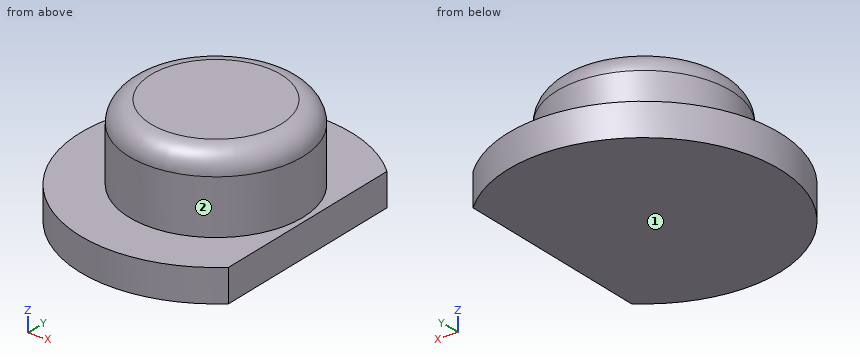
```python
from build123d import *

# Parameters (mm, degrees)
BOX116_W          = 10
BOX116_H          = 10
BOX116_DEPTH      = 10
CYLINDER019_R     = 4
CYLINDER019_DEPTH = 5
FILLET003_R       = 1
CYLINDER018_R     = 6.25
CYLINDER018_DEPTH = 1.5


with BuildPart() as cube106:
    # Box116 → Box116 (new body)
    with BuildSketch(Plane(origin=(117.3, 9, 0), x_dir=(1, 0, 0), z_dir=(0, 0, 1))):
        with Locations((5, 5)):
            Rectangle(BOX116_W, BOX116_H)
    extrude(amount=BOX116_DEPTH)


with BuildPart() as obj1:
    # Cylinder019 → Cylinder019 (new body)
    with BuildSketch(Plane(origin=(131.07, 14, 6.3), x_dir=(1, 0, 0), z_dir=(0, 0, 1))):
        Circle(CYLINDER019_R)
    extrude(amount=CYLINDER019_DEPTH)

    # Fillet003
    fillet003_edges = [obj1.edges().sort_by_distance(p)[0] for p in [
        (127.07, 14, 11.3),
    ]]
    fillet(fillet003_edges, radius=FILLET003_R)


with BuildPart() as cut072:
    # Cylinder018 → Cylinder018 (new body)
    with BuildSketch(Plane(origin=(131.07, 14, 6.3), x_dir=(1, 0, 0), z_dir=(0, 0, 1))):
        Circle(CYLINDER018_R)
    extrude(amount=CYLINDER018_DEPTH)

    # Fusion014: union obj1
    add(obj1.part)


with BuildPart() as cut072_1:
    # Fusion014 placement: moved
    add(cut072.part.moved(Location((-18, 0, 0))))

    # Cut072: cut Cube106
    add(cube106.part, mode=Mode.SUBTRACT)


solid = cut072_1.part
```
Read the model definition and answer for the solid it produces. Units are mm, in the model's axes. Face numbers are marked on the shaded views. A direction names the side the tool comes from. Coordinates: 2 decimals unless noted, no trailing zeros. Loops run counter-clockwise (first coordinate to the right, second up) from the corner with the lowest first, then second, coordinate; pieces in that order, holes last. Notation, with made-up numbers: (10, 52.25) -> (34, 52.25) arc R15 ccw to (34, 70.25) -> close; hole circle Ø10 at (7, 69). An arc over 180 degrees is marked (long way). Return JSON: item names as keys, results as strings.
Item 1: Find the intervals of material crossed by probe 1 along Z at (x, y) = (110.5, 17.75); probe 2 along Y at (x, z) = (116.5, 10.2); probe 3 along X at (y, z) = (18.5, 7.6), in increasing order.
Answers:
{"probe 1": "z = 6.3 to 7.8", "probe 2": "y = 11.94 to 16.06", "probe 3": "x = 108.73 to 117.3"}
Item 2: Find section D-D (y = 18.25). Determine the outline of the cut face in (x, z), plus the area to 3 significant figures.
Answers:
{"outline": "(108.49, 6.3) -> (117.3, 6.3) -> (117.3, 7.8) -> (108.49, 7.8) -> close", "area": "13.2 mm2"}
Item 3: Find section A-A (y = 14). Determine the outline of the cut face in (x, z).
Answers:
{"outline": "(106.82, 6.3) -> (117.3, 6.3) -> (117.3, 7.8) -> (117.07, 7.8) -> (117.07, 10.3) arc R1 ccw to (116.07, 11.3) -> (110.07, 11.3) arc R1 ccw to (109.07, 10.3) -> (109.07, 7.8) -> (106.82, 7.8) -> close"}
Item 4: Flat-ended cylindrical pins translate along their axes: P1, Ø1.5, axis at x = 116, z = 10, coming from the -Y side; P2, Ø1, axis at y = 14, z = 9, coming from the -X side. Find the tip coordinate at first contact, or state that the pin passes through.
Answers:
{"P1": "stops at y = 10.65", "P2": "stops at x = 109.07"}
Item 5: Find section C-C (z = 7.55). Determine the outline of the cut face in (x, y), plus the area to 3 significant figures.
Answers:
{"outline": "(117.3, 9.4) -> (117.3, 18.6) arc R6.25 ccw (long way) to start", "area": "110 mm2"}
Item 6: For the marked faces 1 and 2, determine the directions among +Z, -Z, +X, -X, +Y, -Y from which every point of the face is accessible in a straight line to the end or side of a thin tool.
Answers:
{"face 1": "-Z, +X, -X, +Y, -Y", "face 2": "+Z"}
Item 7: Find section B-B (x = 113.07). Determine the outline of the cut face in (y, z).
Answers:
{"outline": "(7.75, 6.3) -> (20.25, 6.3) -> (20.25, 7.8) -> (18, 7.8) -> (18, 10.3) arc R1 ccw to (17, 11.3) -> (11, 11.3) arc R1 ccw to (10, 10.3) -> (10, 7.8) -> (7.75, 7.8) -> close"}
